Verification items for the finished model (mm, model axes). Face numbers are marked on the shaded views. Give positions to 0.01 mm unless a question says otherwise; leave off trailing zeros. Loops run counter-clockwise (first coordinate to the right, second up) from the corner with the lowest first, then second, coordinate; pieces in that order, holes last. Notation, with made-up numbers: (57.25, -38.75) - (95.25, -38.75) arc R33 cw to (95.25, -0.75) - close; hole circle Ø1 at (-1, 61.25). An arc over 180 degrees is marked (long way). Answer in a Markdown table with one row per item.
```python
from build123d import *


with BuildPart() as part:
    # Эскиз1 → Повернуть1 (revolve)
    with BuildSketch(Plane.XY, mode=Mode.PRIVATE) as revolve_1_sk:
        with BuildLine():
            Line((3.82, -1.2), (2, -1.2))
            Line((2, -1.2), (2, -3.7))
            ThreePointArc((2, -3.7), (3.2, -4.9), (2, -6.1))
            Line((2, -6.1), (0, -6.1))
            Line((0, -6.1), (0, -0.2))
            Line((0, -0.2), (1.25, -0.2))
            Line((1.25, -0.2), (1.25, -0.072764031))
            ThreePointArc((1.25, -0.072764031), (2.554325985, -0.307196852), (3.82, -0.7))
            Line((3.82, -0.7), (3.82, -1.2))
        make_face()
    revolve(revolve_1_sk.sketch.rotate(Axis((0, -0.2, 0), (0, -1, 0)), 180), axis=Axis((0, -0.2, 0), (0, -1, 0)))


solid = part.part
```
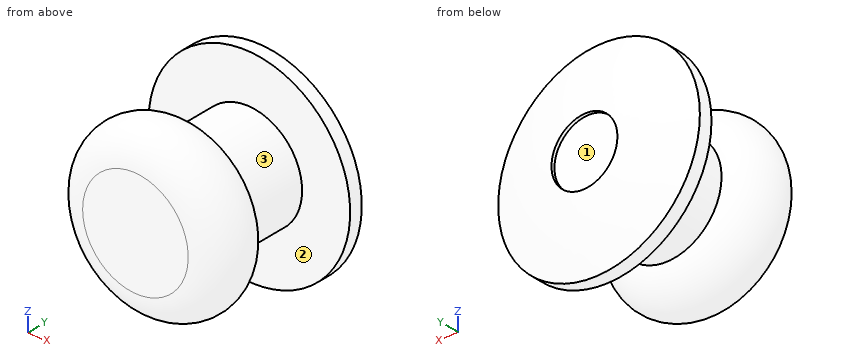
Q1. Sectioned sample at C-C (y = -2.75). Record the cut outline in (x, z), and give its area (3 significant figures).
Completed:
| item | result |
|---|---|
| outline | circle Ø4 at (0, 0) |
| area | 12.6 mm^2 |
Q2. Draft check along X on the marked faces 1, 2 and 3. Enter one of: +X half, -X half, draft (parallel to the pull), parting line (faces both ways), or undercut.
Completed:
| item | result |
|---|---|
| face 1 | undercut |
| face 2 | draft |
| face 3 | parting line |
Q3. Sectioned sample at B-B (z = 0). Record the cut outline in (x, y).
Completed:
| item | result |
|---|---|
| outline | (-3.82, -1.2) - (-2, -1.2) - (-2, -3.7) arc R1.2 ccw to (-2, -6.1) - (2, -6.1) arc R1.2 ccw to (2, -3.7) - (2, -1.2) - (3.82, -1.2) - (3.82, -0.7) arc R10.77 ccw to (1.25, -0.07) - (1.25, -0.2) - (-1.25, -0.2) - (-1.25, -0.07) arc R10.77 ccw to (-3.82, -0.7) - close |
Q4. Sectioned sample at A-A (x = 0). Record the cut outline in (y, z), and give its area (3 significant figures).
Completed:
| item | result |
|---|---|
| outline | (-6.1, -2) arc R1.2 ccw to (-3.7, -2) - (-1.2, -2) - (-1.2, -3.82) - (-0.7, -3.82) arc R10.77 ccw to (-0.07, -1.25) - (-0.2, -1.25) - (-0.2, 1.25) - (-0.07, 1.25) arc R10.77 ccw to (-0.7, 3.82) - (-1.2, 3.82) - (-1.2, 2) - (-3.7, 2) arc R1.2 ccw to (-6.1, 2) - close |
| area | 31.1 mm^2 |
Q5. Go/stop test with flat-tipped pins: P1, Ø1, axis at x = 1, y = -5.5, coming from the +Z side; P2, Ø2, axis at y = -5, z = 1, coming from the -X side. Record where each tip stops, or that it passes through.
Completed:
| item | result |
|---|---|
| P1 | z = 3.11 |
| P2 | x = -3.2 |
Q6. Thickness scan on line 1 (Y direction, x = -0.5, z = 0.5); line 2 (Y direction, x = -1.25, z = 1.75); line 3 (Y direction, x = 1, z = 2.5). Record the ranges inside material, lowest first.
Completed:
| item | result |
|---|---|
| line 1 | -6.1 to -0.2 |
| line 2 | -6.09 to -3.71, -1.2 to -0.22 |
| line 3 | -5.88 to -3.92, -1.2 to -0.34 |
Q7. Sectioned sample at D-D (y = -0.5). Record the cut outline in (x, z).
Completed:
| item | result |
|---|---|
| outline | circle Ø6.49 at (0, 0) |
